from build123d import *
from build123d.topology import SkipClean

# Parameters (mm, degrees)
SKETCH_1_R          = 3
SKETCH_1_R_2        = 1.5
EXTRUDE_1_DEPTH     = 8
EXTRUDE_START       = 8
SKETCH_2_R          = 10
SKETCH_2_R_2        = 1.5
SKETCH_2_R_3        = 3
EXTRUDE_2_DEPTH     = 8
CUT_EXTRUDE_START   = -5
SKETCH_3_R          = 35
SKETCH_3_R_2        = 4
SKETCH_3_R_3        = 11
CUT_EXTRUDE_2_DEPTH = 5
CHAMFER_1_SIZE      = 3
CUT_EXTRUDE_START_2 = -2
SKETCH_3_4_R        = 4
CUT_EXTRUDE_3_DEPTH = 2


with BuildPart() as part:
    # Sketch 1 → Extrude 1 (new body)
    with BuildSketch(Plane(origin=(0, 0, 0), x_dir=(1, 0, 0), z_dir=(0, 1, 0))):
        with BuildLine():
            ThreePointArc((0, 80), (32.794915451, 57.226754294), (22.912878475, 18.542486889))
            ThreePointArc((22.912878475, 18.542486889), (21.922333534, 12.656865167), (27.514703933, 10.571891388))
            ThreePointArc((27.514703933, 10.571891388), (65.95728072, -0.212147251), (69.282032303, -40))
            ThreePointArc((69.282032303, -40), (33.162365269, -57.014607042), (4.601825458, -29.114378278))
            ThreePointArc((4.601825458, -29.114378278), (0, -25.313730334), (-4.601825458, -29.114378278))
            ThreePointArc((-4.601825458, -29.114378278), (-33.162365269, -57.014607042), (-69.282032303, -40))
            ThreePointArc((-69.282032303, -40), (-65.95728072, -0.212147251), (-27.514703933, 10.571891388))
            ThreePointArc((-27.514703933, 10.571891388), (-21.922333534, 12.656865167), (-22.912878475, 18.542486889))
            ThreePointArc((-22.912878475, 18.542486889), (-32.794915451, 57.226754294), (0, 80))
        make_face()
        with Locations(Location((0, 0, 0), (0, 0, 270))):
            Circle(SKETCH_1_R, mode=Mode.SUBTRACT)
        with Locations(Location((0, 7, 0), (0, 0, 270))):
            Circle(SKETCH_1_R_2, mode=Mode.SUBTRACT)
        with Locations(Location((7, 0, 0), (0, 0, 270))):
            Circle(SKETCH_1_R_2, mode=Mode.SUBTRACT)
        with Locations(Location((0, -7, 0), (0, 0, 270))):
            Circle(SKETCH_1_R_2, mode=Mode.SUBTRACT)
        with Locations(Location((-7, 0, 0), (0, 0, 270))):
            Circle(SKETCH_1_R_2, mode=Mode.SUBTRACT)
        with Locations(Location((0, 55, 0), (0, 0, 270))):
            Circle(SKETCH_1_R_2, mode=Mode.SUBTRACT)
        with Locations(Location((0, 35, 0), (0, 0, 270))):
            Circle(SKETCH_1_R_2, mode=Mode.SUBTRACT)
        with Locations(Location((47.631397208, -27.5, 0), (0, 0, 270))):
            Circle(SKETCH_1_R_2, mode=Mode.SUBTRACT)
        with Locations(Location((30.310889132, -17.5, 0), (0, 0, 270))):
            Circle(SKETCH_1_R_2, mode=Mode.SUBTRACT)
        with Locations(Location((-47.631397208, -27.5, 0), (0, 0, 270))):
            Circle(SKETCH_1_R_2, mode=Mode.SUBTRACT)
        with Locations(Location((-30.310889132, -17.5, 0), (0, 0, 270))):
            Circle(SKETCH_1_R_2, mode=Mode.SUBTRACT)
    extrude(amount=EXTRUDE_1_DEPTH)

    # Sketch 2 → Extrude 2 (add)
    with SkipClean():  # the faces are left unmerged after this step: merging them gives an invalid solid
        with BuildSketch(Plane.XZ.offset(EXTRUDE_START)):
            with Locations(Location((0, 0, 0), (0, 0, 90))):
                Circle(SKETCH_2_R)
            with Locations(Location((-7, 0, 0), (0, 0, 270))):
                Circle(SKETCH_2_R_2, mode=Mode.SUBTRACT)
            with Locations(Location((0, -7, 0), (0, 0, 270))):
                Circle(SKETCH_2_R_2, mode=Mode.SUBTRACT)
            with Locations(Location((7, 0, 0), (0, 0, 270))):
                Circle(SKETCH_2_R_2, mode=Mode.SUBTRACT)
            with Locations(Location((0, 7, 0), (0, 0, 270))):
                Circle(SKETCH_2_R_2, mode=Mode.SUBTRACT)
            with Locations(Location((0, 0, 0), (0, 0, 270))):
                Circle(SKETCH_2_R_3, mode=Mode.SUBTRACT)
        extrude(amount=-EXTRUDE_2_DEPTH)

    # Sketch 3 → Cut-Extrude 2 (cut)
    # profile 1 of 4: a face of its own
    with SkipClean():  # the faces are left unmerged after this step: merging them gives an invalid solid
        with BuildSketch(Plane(origin=(0, 8, 0), x_dir=(1, 0, 0), z_dir=(0, 1, 0)).offset(CUT_EXTRUDE_START)):
            with Locations((0, 45)):
                Circle(SKETCH_3_R)
            with Locations(Location((0, 45, 0), (0, 0, 270))):
                Circle(SKETCH_3_R_2, mode=Mode.SUBTRACT)
        # profile 2 of 4: a face of its own
        with BuildSketch(Plane(origin=(0, 8, 0), x_dir=(1, 0, 0), z_dir=(0, 1, 0)).offset(CUT_EXTRUDE_START)):
            with Locations((38.97114317, -22.5)):
                Circle(SKETCH_3_R)
            with Locations(Location((38.97114317, -22.5, 0), (0, 0, 270))):
                Circle(SKETCH_3_R_2, mode=Mode.SUBTRACT)
        # profile 3 of 4: a face of its own
        with BuildSketch(Plane(origin=(0, 8, 0), x_dir=(1, 0, 0), z_dir=(0, 1, 0)).offset(CUT_EXTRUDE_START)):
            with Locations((-38.97114317, -22.5)):
                Circle(SKETCH_3_R)
            with Locations(Location((-38.97114317, -22.5, 0), (0, 0, 270))):
                Circle(SKETCH_3_R_2, mode=Mode.SUBTRACT)
        # profile 4 of 4: a face of its own
        with BuildSketch(Plane(origin=(0, 8, 0), x_dir=(1, 0, 0), z_dir=(0, 1, 0)).offset(CUT_EXTRUDE_START)):
            Circle(SKETCH_3_R_3)
        extrude(amount=CUT_EXTRUDE_2_DEPTH, mode=Mode.SUBTRACT)

    # Chamfer 1
    chamfer_1_edges = [part.edges().sort_by_distance(p)[0] for p in [
        (0, 0, -10),
    ]]
    chamfer(chamfer_1_edges, length=CHAMFER_1_SIZE)

    # Sketch 3_4 → Cut-Extrude 3 (cut)
    with SkipClean():  # the faces are left unmerged after this step: merging them gives an invalid solid
        with BuildSketch(Plane(origin=(0, 8, 0), x_dir=(1, 0, 0), z_dir=(0, 1, 0)).offset(CUT_EXTRUDE_START_2)):
            with Locations(Location((-38.97114317, -22.5, 0), (0, 0, 270))):
                Circle(SKETCH_3_4_R)
            with Locations(Location((38.97114317, -22.5, 0), (0, 0, 270))):
                Circle(SKETCH_3_4_R)
            with Locations(Location((0, 45, 0), (0, 0, 270))):
                Circle(SKETCH_3_4_R)
        extrude(amount=CUT_EXTRUDE_3_DEPTH, mode=Mode.SUBTRACT)


solid = part.part
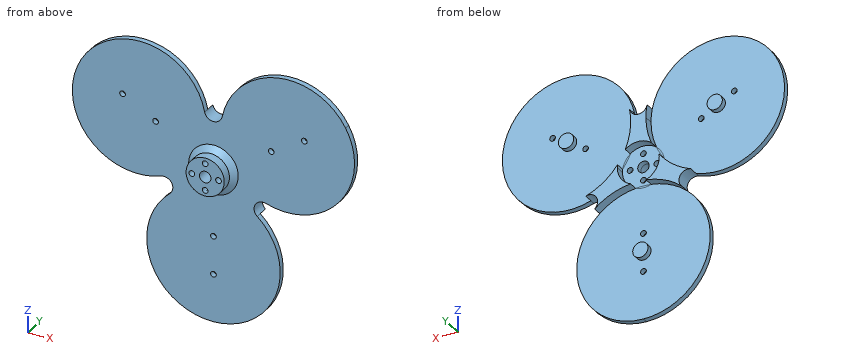
Geometry: final body of the model. Coordinates: model frame, mm. Give positions to 0.01 mm unless a question says otherwise; leave off trailing zeros. Loops run counter-clockwise (first coordinate to the right, second up) from the corner with the lowest first, then second, coordinate; pieces in that order, holes last. Notation, with made-up numbers: (52.25, -31) - (111.25, -31) arc R10 ccw to (111.25, -12) - close; hole circle Ø10 at (5, 18). An arc over 180 degrees is marked (long way). One line per question, with ' | ' between items. Start each with the question number.
(1) Contact query for flat-ended pins moving along their axis: pin 1 (2 mm diameter, centred on y = 2, z = 0, fed in from +X); pin 2 (3 mm diameter, centred on y = -0.5, z = 6.5, fed in from -X); pin 3 (4.5 mm diameter, centred on x = 9, z = 6.5, fed in from +Y); pin 4 (2.5 mm diameter, centred on x = 0, z = -35, fed in from +Y). Output: stop coordinate, or through.
(2) Section query B-B on z = -45. Return loops of the section in (x, y).
(3) Ray query, line 1 (Z direction, x = 0, y = 1.75); line 2 (X direction, y = -4, z = 0); line 3 (X direction, y = 1.6, z = 0). Return the intervals inside material, ascending. Write a range as from..to.
(4) Section query C-C on z = 45.5. Return loops of the section in (x, y), then the cut area to 3 significant figures.
The answers:
1) pin 1: x = 66.59 | pin 2: x = -70.79 | pin 3: y = 3 | pin 4: through
2) outline: (-35, 0) - (35, 0) - (35, 3) - (4, 3) - (4, 6) - (-4, 6) - (-4, 3) - (-35, 3) - close
3) line 1: -80..-56.5, -53.5..-36.5, -33.5..-8.5, -5.5..-3, 3..5.5, 8.5..25.31 | line 2: -10..-8.5, -5.5..-3, 3..5.5, 8.5..10 | line 3: -65.78..-8.5, -5.5..-3, 3..5.5, 8.5..65.78
4) outline: (-65.35, 0) - (-12.59, 0) - (-12.59, 3) - (-65.35, 3) - close; (12.59, 0) - (65.35, 0) - (65.35, 3) - (12.59, 3) - close | area: 317 mm2
